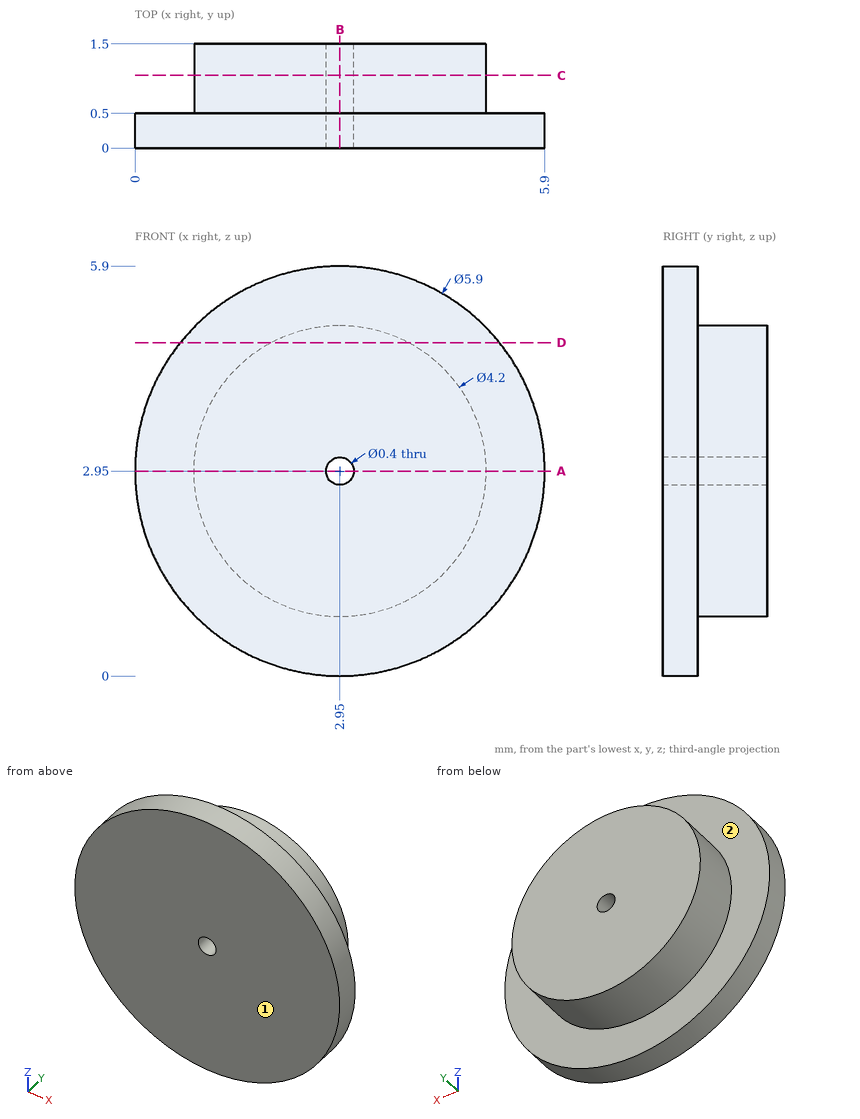
Can you work these out from the drawing? Everything is in mm from the part's minimum corner. A direction names the side the tool comes from. Round coordinates to 2 decimals unless told otherwise and drop trailing zeros. Order: outer loops, then holes, each group sorted by start corner. A loop starts at its lowest first (then second) coordinate and runs counter-clockwise, first axis right, second up. Notation, with made-up numbers: (-38, 0.25) -> (-14, 0.25) arc R13 ccw to (-14, 20.25) -> close; hole circle Ø5 at (-30, 55.25). An arc over 180 degrees is marked (long way). Use CSV: the item, a comma, the result in double quotes.
1. Which directions (+Z, -Z, +X, -X, +Y, -Y) give clear straight access to the entire face, cutting with the end or side of a thin tool? Please do the marked faces 1 and 2.
Recorded:
face 1,"+Z, -Z, +X, -X, -Y"
face 2,"+Y"
2. I want a section at B-B on x = 2.95. List the corners of the cut face in (y, z) for me.
Recorded:
outline,"(0, 0) -> (0.5, 0) -> (0.5, 0.85) -> (1.5, 0.85) -> (1.5, 2.75) -> (0, 2.75) -> close; (0, 3.15) -> (1.5, 3.15) -> (1.5, 5.05) -> (0.5, 5.05) -> (0.5, 5.9) -> (0, 5.9) -> close"
3. I want a section at C-C on y = 1.05. List the corners of the cut face in (x, z) for me, and give its area (3 significant figures).
Recorded:
outline,"circle Ø4.2 at (2.95, 2.95); hole circle Ø0.4 at (2.95, 2.95)"
area,"13.7 mm2"
4. I want a section at D-D on z = 4.8. List the corners of the cut face in (x, y) for me, and give its area (3 significant figures).
Recorded:
outline,"(0.65, 0) -> (5.25, 0) -> (5.25, 0.5) -> (3.94, 0.5) -> (3.94, 1.5) -> (1.96, 1.5) -> (1.96, 0.5) -> (0.65, 0.5) -> close"
area,"4.29 mm2"
5. I need wall thicknesses on line 1 along X through (y, z) = (0.4, 2.95); line 2 along X through (y, z) = (1.1, 2.95); line 3 along Y through (x, z) = (4.95, 1.8). Which ranges of each line are inside material? Lowest first, please.
Recorded:
line 1,"x = 0 to 2.75, 3.15 to 5.9"
line 2,"x = 0.85 to 2.75, 3.15 to 5.05"
line 3,"y = 0 to 0.5"
6. I want a section at A-A on z = 2.95. List the corners of the cut face in (x, y) for me.
Recorded:
outline,"(0, 0) -> (2.75, 0) -> (2.75, 1.5) -> (0.85, 1.5) -> (0.85, 0.5) -> (0, 0.5) -> close; (3.15, 0) -> (5.9, 0) -> (5.9, 0.5) -> (5.05, 0.5) -> (5.05, 1.5) -> (3.15, 1.5) -> close"
